Model file for the job. Use its own axes, mm. Coordinates: 2 decimals unless noted, no trailing zeros. Order: outer loops, then holes, each group sorted by start corner. A loop starts at its lowest first (then second) coordinate and runs counter-clockwise, first axis right, second up. Notation, with made-up numbers: (77.25, 16.25) -> (89.25, 16.25) arc R28 ccw to (89.25, 55.25) -> close; hole circle Ø7 at (-17.75, -2.75). An arc over 180 degrees is marked (long way). Return JSON: item names as keys, results as strings. Group by question number.
1) Cut at A-A (y = 50.8). Write the cut outline in (x, z) (3 decimals).
2) Probe line 1 (Y direction, x = 1.5, z = -40); line 2 (Y direction, x = -2.5, z = -56); line 3 (Z direction, x = 2.5, y = 114). List the from-to ranges inside material, lowest first.
3) Cut at C-C (x = -2). Write the cut outline in (y, z), and give its area (3 significant figures).
4) Cut at D-D (z = 29). Write the cut outline in (x, y) (3 decimals).
5) Cut at B-B (z = -49.5). Write the cut outline in (x, y) (3 decimals).
6) Pull direction Z, two halves, no side cores. Call faces 1 (the cylindrical face through (0, 43.1, -40.7)), 2 (the flat face through (0, 127, 2)), 3 (the flat face through (0, -2, -127)): +Z half, -Z half, draft (parallel to the pull), parting line (faces both ways), or undercut.
7) Flat gauge pins, fed straight in: pin 1 (20.5 mm diameter, centred on y = 50.8, z = -50.8, fed in from -X); pin 2 (1.5 mm diameter, centred on x = 0.5, z = 32, fed in from -Y); pin 3 (3 mm diameter, centred on x = 1.5, y = 27, fed in from +Z). Where does each tip first touch, or does it go through?
from build123d import *

# Parameters (mm, degrees)
SKETCH1_W           = 254
SKETCH1_H           = 254
BOSS_EXTRUDE1_DEPTH = 3.175
FILLET1_R           = 241.3
CUT_EXTRUDE1_REACH  = 8.35
SKETCH2_R           = 12.7


with BuildPart() as part:
    # Sketch1 → Boss-Extrude1 (new body, symmetric)
    with BuildSketch(Plane(origin=(0, 0, 0), x_dir=(0, 0, -1), z_dir=(1, 0, 0))):
        Rectangle(SKETCH1_W, SKETCH1_H)
    extrude(amount=BOSS_EXTRUDE1_DEPTH, both=True)

    # Fillet1
    fillet1_edges = [part.edges().sort_by_distance(p)[0] for p in [
        (0, -127, 127),
    ]]
    fillet(fillet1_edges, radius=FILLET1_R)

    # Sketch2 → Cut-Extrude1 (cut, up to next)
    with BuildSketch(Plane(origin=(3.175, 0, 0), x_dir=(0, 0, -1), z_dir=(1, 0, 0)), mode=Mode.PRIVATE) as cut_extrude1_sk1:
        with Locations((50.8, 50.8)):
            Circle(SKETCH2_R)
    cut_extrude1_tool1 = extrude(cut_extrude1_sk1.sketch, amount=-CUT_EXTRUDE1_REACH, mode=Mode.PRIVATE) & part.part
    add(cut_extrude1_tool1.solids().sort_by_distance((3.175, 50.8, -50.8))[0], mode=Mode.SUBTRACT)


solid = part.part
Answers below:
{
 "1": {"outline": "(-3.175, -127) -> (3.175, -127) -> (3.175, -63.5) -> (-3.175, -63.5) -> close; (-3.175, -38.1) -> (3.175, -38.1) -> (3.175, 118.495) -> (-3.175, 118.495) -> close"},
 "2": {"line 1": "y = -115.28 to 44.12, 57.48 to 127", "line 2": "y = -119.85 to 39.21, 62.39 to 127", "line 3": "z = -127 to 127"},
 "3": {"outline": "(-127, -127) -> (127, -127) -> (127, 127) -> (114.3, 127) arc R241.3 ccw to (-127, -114.3) -> close; hole circle Ø25.4 at (50.8, -50.8)", "area": "51,500 mm^2"},
 "4": {"outline": "(-3.175, -79.841) -> (3.175, -79.841) -> (3.175, 127) -> (-3.175, 127) -> close"},
 "5": {"outline": "(-3.175, -118.136) -> (3.175, -118.136) -> (3.175, 38.167) -> (-3.175, 38.167) -> close; (-3.175, 63.433) -> (3.175, 63.433) -> (3.175, 127) -> (-3.175, 127) -> close"},
 "6": {"face 1": "undercut", "face 2": "draft", "face 3": "-Z half"},
 "7": {"pin 1": "passes through", "pin 2": "stops at y = -78.16", "pin 3": "stops at z = 111.23"}
}
